Read the model definition and answer for the solid it produces. Units are mm, in the model's axes. Give positions to 0.01 mm unless a question says otherwise; leave off trailing zeros. Loops run counter-clockwise (first coordinate to the right, second up) from the corner with the lowest first, then second, coordinate; pieces in that order, holes last. Notation, with made-up numbers: (50, -28) - (98, -28) arc R26 ccw to (98, 9) - close; hole circle Ø10 at (-10, 80.25). An arc over 180 degrees is marked (long way). Write item = value, one per line.
Autodesk Inventor part; units mm, degrees
ref_plane "YZ Plane" through (0, 0, 0) normal (1, 0, 0) x (0, 1, 0)
ref_plane "XZ Plane" through (0, 0, 0) normal (0, 1, 0) x (-1, 0, 0)
ref_plane "XY Plane" through (0, 0, 0) normal (0, 0, 1) x (1, 0, 0)
sketch "Boceto1" plane through (0, 0, 0) normal (0, 1, 0) x (-1, 0, 0)
  line L0 (-105.368, 99.7227) -> (81.632, 99.7227)
  line L1 (81.632, 99.7227) -> (81.632, -87.2773)
  line L2 (81.632, -87.2773) -> (-105.368, -87.2773)
  line L3 (-105.368, -87.2773) -> (-105.368, 99.7227)
  line L4 (-89.368, 74.7227) -> (-85.368, 74.7227)
  line L5 (-85.368, 74.7227) -> (-85.368, 55.7227)
  line L6 (-85.368, 55.7227) -> (-89.368, 55.7227)
  line L7 (-89.368, 55.7227) -> (-89.368, 74.7227)
  line L8 (-89.368, -62.2773) -> (-85.368, -62.2773)
  line L9 (-85.368, -62.2773) -> (-85.368, -43.2773)
  line L10 (-85.368, -43.2773) -> (-89.368, -43.2773)
  line L11 (-89.368, -43.2773) -> (-89.368, -62.2773)
  line L12 (-47.368, 64.7227) -> (23.632, 64.7227)
  line L13 (23.632, 64.7227) -> (23.632, 40.7227)
  line L14 (23.632, 40.7227) -> (-47.368, 40.7227)
  line L15 (-47.368, 40.7227) -> (-47.368, 64.7227)
  circle A0 centre (-49.368, 67.7227) radius 1.5
  line L16 (-51.868, 70.2227) -> (28.132, 70.2227)
  line L17 (28.132, 70.2227) -> (28.132, 34.2227)
  line L18 (28.132, 34.2227) -> (-51.868, 34.2227)
  line L19 (-51.868, 34.2227) -> (-51.868, 70.2227)
  circle A1 centre (25.632, 67.7227) radius 1.5
  circle A2 centre (-49.368, 36.7227) radius 1.5
  circle A3 centre (25.632, 36.7227) radius 1.5
  line L20 (3.632, -29.2773) -> (16.632, -29.2773)
  line L21 (16.632, -29.2773) -> (16.632, -42.2773)
  line L22 (16.632, -42.2773) -> (3.632, -42.2773)
  line L23 (3.632, -42.2773) -> (3.632, -29.2773)
  line L24 (-11.968, -6.7773) -> (-8.468, -6.7773)
  line L25 (-8.468, -6.7773) -> (-8.468, -13.2773)
  line L26 (-8.468, -13.2773) -> (-11.968, -13.2773)
  line L27 (-11.968, -13.2773) -> (-11.968, -6.7773)
  line L28 (32.232, -6.7773) -> (28.732, -6.7773)
  line L29 (28.732, -6.7773) -> (28.732, -13.2773)
  line L30 (28.732, -13.2773) -> (32.232, -13.2773)
  line L31 (32.232, -13.2773) -> (32.232, -6.7773)
  line L32 (65.632, 74.7227) -> (61.632, 74.7227)
  line L33 (61.632, 74.7227) -> (61.632, 55.7227)
  line L34 (61.632, 55.7227) -> (65.632, 55.7227)
  line L35 (65.632, 55.7227) -> (65.632, 74.7227)
  line L36 (65.632, -43.2773) -> (65.632, -62.2773)
  line L37 (65.632, -62.2773) -> (61.632, -62.2773)
  line L38 (61.632, -62.2773) -> (61.632, -43.2773)
  line L39 (61.632, -43.2773) -> (65.632, -43.2773)
  point P0 (0, 0)
  dimension "d0" = 187
  dimension "d1" = 187
  dimension "d2" = 16
  dimension "d3" = 25
  dimension "d4" = 19
  dimension "d5" = 4
  dimension "d7" = 71
  dimension "d8" = 58
  dimension "d10" = 3
  dimension "d11" = 36
  dimension "d12" = 80
  dimension "d13" = 4.5
  dimension "d14" = 5.5
  dimension "d15" = 2.5
  dimension "d16" = 2.5
  dimension "d17" = 35
  dimension "d26" = 16
  dimension "d27" = 25
  dimension "d28" = 4
  dimension "d29" = 19
  dimension "d30" = 2.5
  dimension "d31" = 2.5
  dimension "d32" = 2.5
  dimension "d33" = 2.5
  dimension "d34" = 2.5
  dimension "d35" = 2.5
  dimension "d36" = 13
  dimension "d37" = 13
  dimension "d38" = 65
  dimension "d39" = 45
  dimension "d40" = 6.5
  dimension "d41" = 3.5
  dimension "d42" = 29
  dimension "d45" = 29
  dimension "d46" = 3.5
  dimension "d47" = 6.5
  dimension "d48" = 16
  dimension "d49" = 19
  dimension "d50" = 4
  dimension "d51" = 25
  dimension "d52" = 16
  dimension "d53" = 4
  dimension "d54" = 19
  dimension "d55" = 25
  dimension "d72" = 37.2
  dimension "d73" = 12.1
  dimension "d74" = 24
extrude "Extrusión1" add sketch "Boceto1" along normal blind 3 contours L0 L1 L2 L3 | L16 L17 L18 L19
sketch "Boceto2" plane through (0, 3, 0) normal (0, 1, 0) x (1, 0, 0)
  line L0 (-16.632, 29.2773) -> (-16.632, 42.2773)
  line L1 (-16.632, 42.2773) -> (-3.632, 42.2773)
  line L2 (-3.632, 42.2773) -> (-3.632, 29.2773)
  line L3 (-3.632, 29.2773) -> (-16.632, 29.2773)
  line L4 (3.368, 22.2773) -> (-23.632, 22.2773)
  line L5 (-23.632, 22.2773) -> (-23.632, 49.2773)
  line L6 (-23.632, 49.2773) -> (3.368, 49.2773)
  line L7 (3.368, 49.2773) -> (3.368, 22.2773)
  circle A0 centre (-0.132, 25.7773) radius 1.5
  line L8 (-10.132, 22.2773) -> (-10.132, 49.2773)
  line L9 (3.368, 35.7773) -> (-23.632, 35.7773)
  circle A1 centre (-20.132, 25.7773) radius 1.5
  circle A2 centre (-0.132, 45.7773) radius 1.5
  circle A3 centre (-20.132, 45.7773) radius 1.5
  point P0 (0, 0)
  dimension "d58" = 7
  dimension "d59" = 7
  dimension "d60" = 7
  dimension "d61" = 7
  dimension "d62" = 3
  dimension "d63" = 3.5
  dimension "d64" = 3.5
  dimension "d75" = 3.5
extrude "Extrusión2" cut sketch "Boceto2" against normal through all contours A0 | A1 | A2 | A3
sketch "Boceto3" plane through (0, 3, 0) normal (0, 1, 0) x (1, 0, 0)
  line L0 (-81.632, -99.7227) -> (105.368, -99.7227)
  line L1 (-81.632, 87.2773) -> (-81.632, -99.7227)
  circle A0 centre (11.868, -19.7227) radius 4.75
  point P0 (0, 0)
  dimension "d67" = 9.5
  dimension "d68" = 93.5
  dimension "d69" = 80
extrude "Extrusión3" cut sketch "Boceto3" against normal through all
properties part number "Tapa final"
1) The mould has two halves that part along Z. Classify faces 1 (the face through (16.4, 1.5, 18.3)), 2 (the face through (13, 0, 8)): pulls with the +Z half, pulls with the -Z half, needs draft (parallel to the pull), parting line crosses it, or undercut.
Output:
face_1 = undercut
face_2 = needs draft
2) A cutting plane is placed at A-A on x = -14.5. Determine the outline of the cut face in (y, z), then the cut area to 3 significant figures.
Output:
outline = (0, -87.28) - (3, -87.28) - (3, -42.28) - (0, -42.28) - close; (0, -29.28) - (3, -29.28) - (3, 40.72) - (0, 40.72) - close; (0, 64.72) - (3, 64.72) - (3, 99.72) - (0, 99.72) - close
area = 450 mm²
3) Find the intervals of material crossed by probe 1 along X at (y, z) = (2.85, 69.5); probe 2 along Z at (x, y) = (49, 1.4); probe 3 along Z at (x, y) = (-13.5, 0.4), in increasing order.
Output:
probe_1 = -81.63 to -65.63, -61.63 to 85.37, 89.37 to 105.37
probe_2 = -87.28 to 35.27, 38.18 to 66.27, 69.18 to 99.72
probe_3 = -87.28 to -42.28, -29.28 to 40.72, 64.72 to 99.72
4) A cutting plane is placed at C-C on z = -35. Determine the outline of the cut face in (x, y), then the cut area to 3 significant figures.
Output:
outline = (-81.63, 0) - (-16.63, 0) - (-16.63, 3) - (-81.63, 3) - close; (-3.63, 0) - (105.37, 0) - (105.37, 3) - (-3.63, 3) - close
area = 522 mm²
5) A cutting plane is placed at D-D on z = 46.5. Determine the outline of the cut face in (x, y), then the cut area to 3 significant figures.
Output:
outline = (-81.63, 0) - (-23.63, 0) - (-23.63, 3) - (-81.63, 3) - close; (47.37, 0) - (105.37, 0) - (105.37, 3) - (47.37, 3) - close
area = 348 mm²
6) A cutting plane is placed at B-B on z = -60. Determine the outline of the cut face in (x, y), then the cut area to 3 significant figures.
Output:
outline = (-81.63, 0) - (-65.63, 0) - (-65.63, 3) - (-81.63, 3) - close; (-61.63, 0) - (85.37, 0) - (85.37, 3) - (-61.63, 3) - close; (89.37, 0) - (105.37, 0) - (105.37, 3) - (89.37, 3) - close
area = 537 mm²
